from build123d import *

# Parameters (mm, degrees)
SKETCH_1_R          = 1.6
SKETCH_1_R_2        = 3.5
EXTRUDE_1_DEPTH     = 5
SKETCH_3_R          = 1.6
EXTRUDE_3_DEPTH     = 5
EXTRUDE_4_DEPTH     = 5
CUT_EXTRUDE_1_DEPTH = 21.9


with BuildPart() as part:
    # 草图1 → 凸台-拉伸1 (new body)
    with BuildSketch(Plane(origin=(0, 0, 0), x_dir=(1, 0, 0), z_dir=(0, 1, 0))):
        with BuildLine():
            Line((30, 23.923257503), (36.791550388, 23.923257503))
            Line((36.791550388, 23.923257503), (45, 23.923257503))
            Line((45, 23.923257503), (45, 18.923257503))
            Line((45, 18.923257503), (30, 18.923257503))
            Line((30, 18.923257503), (7.290296698, 5.071204372))
            ThreePointArc((7.290296698, 5.071204372), (0, 3.023257503), (-7.290296698, 5.071204372))
            Line((-7.290296698, 5.071204372), (-30, 18.923257503))
            Line((-30, 18.923257503), (-45, 18.923257503))
            Line((-45, 18.923257503), (-45, 23.923257503))
            Line((-45, 23.923257503), (-36.791550388, 23.923257503))
            Line((-36.791550388, 23.923257503), (-30, 23.923257503))
            Line((-30, 23.923257503), (-3.410329214, 30.601536284))
            ThreePointArc((-3.410329214, 30.601536284), (0, 31.023257503), (3.410329214, 30.601536284))
            Line((3.410329214, 30.601536284), (30, 23.923257503))
        make_face()
        with Locations((0, 24.023257503)):
            Circle(SKETCH_1_R, mode=Mode.SUBTRACT)
        with Locations((0, 10.023257503)):
            Circle(SKETCH_1_R, mode=Mode.SUBTRACT)
        with Locations((-7, 17.023257503)):
            Circle(SKETCH_1_R, mode=Mode.SUBTRACT)
        with Locations((7, 17.023257503)):
            Circle(SKETCH_1_R, mode=Mode.SUBTRACT)
        with Locations((0, 17.023257503)):
            Circle(SKETCH_1_R_2, mode=Mode.SUBTRACT)
    extrude(amount=EXTRUDE_1_DEPTH)

    # 草图3 → 凸台-拉伸3 (add)
    with BuildSketch(Plane(origin=(0, 0, -23.923257503), x_dir=(-1, 0, 0), z_dir=(0, 0, -1))):
        Polygon((-45, 5), (-63, 5), (-63, -30), (-43, -30), (-43, -20.44669455), (-43, -7.63227787), (-43, 5), align=None)
        with Locations((-58, -9.8)):
            Circle(SKETCH_3_R, mode=Mode.SUBTRACT)
        with Locations((-58, -24.8)):
            Circle(SKETCH_3_R, mode=Mode.SUBTRACT)
        with Locations((-48, -24.8)):
            Circle(SKETCH_3_R, mode=Mode.SUBTRACT)
        with Locations((-48, -9.8)):
            Circle(SKETCH_3_R, mode=Mode.SUBTRACT)
        Polygon((43, -20.44669455), (43, -30), (63, -30), (63, 5), (45, 5), (43, 5), (43, -7.63227787), align=None)
        with Locations((48, -9.8)):
            Circle(SKETCH_3_R, mode=Mode.SUBTRACT)
        with Locations((48, -24.8)):
            Circle(SKETCH_3_R, mode=Mode.SUBTRACT)
        with Locations((58, -24.8)):
            Circle(SKETCH_3_R, mode=Mode.SUBTRACT)
        with Locations((58, -9.8)):
            Circle(SKETCH_3_R, mode=Mode.SUBTRACT)
    extrude(amount=-EXTRUDE_3_DEPTH)

    # 草图5 → 凸台-拉伸4 (add)
    with BuildSketch(Plane(origin=(0, 0, -23.923257503), x_dir=(-1, 0, 0), z_dir=(0, 0, -1))):
        Polygon((14, 0), (43, -13), (43, 0), align=None)
        Polygon((-43, 0), (-14, 0), (-43, -13), align=None)
    extrude(amount=-EXTRUDE_4_DEPTH)

    # 草图6 → 切除-拉伸1 (cut, through all)
    with BuildSketch(Plane(origin=(0, 0, -23.923257503), x_dir=(-1, 0, 0), z_dir=(0, 0, -1))):
        Polygon((-63, -2.3), (-30, 5), (-63, 5), align=None)
        Polygon((63, -2.3), (30, 5), (63, 5), align=None)
    extrude(amount=-CUT_EXTRUDE_1_DEPTH, mode=Mode.SUBTRACT)


solid = part.part
Model file for the job. Use its own axes, mm. A direction names the side the tool comes from. Round coordinates to 2 decimals unless told otherwise and drop trailing zeros. Loops run counter-clockwise (first coordinate to the right, second up) from the corner with the lowest first, then second, coordinate; pieces in that order, holes last. Notation, with made-up numbers: (70.5, -5.75) - (84.5, -5.75) arc R15 ccw to (84.5, 16.25) - close; hole circle Ø4 at (44, -3.5). An arc over 180 degrees is marked (long way). Write each question's results on one line, items separated by ' | '.
(1) Saw through at D-D, the plane x = 58. List the corners of the cut face in (y, z).
Answer below:
outline: (-30, -23.92) - (-26.4, -23.92) - (-26.4, -18.92) - (-30, -18.92) - close; (-23.2, -23.92) - (-11.4, -23.92) - (-11.4, -18.92) - (-23.2, -18.92) - close; (-8.2, -23.92) - (-1.19, -23.92) - (-1.19, -18.92) - (-8.2, -18.92) - close
(2) 3-axis set-ups, long thin cutter, end or side, ignore diameter. For faces 4 (the cylindrical face through (6.79, 2.46, -18.61)), 5 (the flat face through (-43, -21, -21)): which of +Z, -Z, +X, -X, +Y, -Y reach the whole face in a straight line?
Answer below:
face 4: +Y, -Y | face 5: +Z, -Z, -Y
(3) Mould opens along X. For faces 1 (the cylindrical face through (-0.048, 2.465, -31.023)), 2 (the cylindrical face through (46.52, -25.41, -21.46)), 3 (the flat face through (-63, -16, -21)) say: released by +X, released by -X, zero draft, split by the parting line, or undercut.
Answer below:
face 1: split by the parting line | face 2: undercut | face 3: released by -X
(4) Pin check, flat tips, straight feed: pin 1 (17.5 mm diameter, centred on x = 36, y = -10.5, fed in from -Z); pin 2 (5 mm diameter, centred on x = 34.5, z = -17.5, fed in from +Y). Stop position of each tip, or through.
Answer below:
pin 1: stops at z = -23.92 | pin 2: stops at y = 4.46
(5) Saw through at B-B, the plane x = 0. List the corners of the cut face in (y, z).
Answer below:
outline: (0, -31.02) - (5, -31.02) - (5, -25.62) - (0, -25.62) - close; (0, -22.42) - (5, -22.42) - (5, -20.52) - (0, -20.52) - close; (0, -13.52) - (5, -13.52) - (5, -11.62) - (0, -11.62) - close; (0, -8.42) - (5, -8.42) - (5, -3.02) - (0, -3.02) - close
(6) Saw through at C-C, the plane y = -24.8. List the corners of the cut face in (x, z), then the cut area to 3 significant figures.
Answer below:
outline: (-63, -23.92) - (-59.6, -23.92) - (-59.6, -18.92) - (-63, -18.92) - close; (-56.4, -23.92) - (-49.6, -23.92) - (-49.6, -18.92) - (-56.4, -18.92) - close; (-46.4, -23.92) - (-43, -23.92) - (-43, -18.92) - (-46.4, -18.92) - close; (43, -23.92) - (46.4, -23.92) - (46.4, -18.92) - (43, -18.92) - close; (49.6, -23.92) - (56.4, -23.92) - (56.4, -18.92) - (49.6, -18.92) - close; (59.6, -23.92) - (63, -23.92) - (63, -18.92) - (59.6, -18.92) - close | area: 136 mm^2
(7) Wall check: L1, parallel to Z at x = 0, y = 1.15; L2, parallel to Y at x = -58, z = -21.3; L3, parallel to X at y = -25, z = -22.5. Give the ranges that are in metal, low to high.
Answer below:
L1: z = -31.02 to -25.62, -22.42 to -20.52, -13.52 to -11.62, -8.42 to -3.02 | L2: y = -30 to -26.4, -23.2 to -11.4, -8.2 to -1.19 | L3: x = -63 to -59.59, -56.41 to -49.59, -46.41 to -43, 43 to 46.41, 49.59 to 56.41, 59.59 to 63
(8) Saw through at A-A, the plane y = -14.5. List the corners of the cut face in (x, z).
Answer below:
outline: (-63, -23.92) - (-43, -23.92) - (-43, -18.92) - (-63, -18.92) - close; (43, -23.92) - (63, -23.92) - (63, -18.92) - (43, -18.92) - close
